from build123d import *

# Parameters (mm, degrees)
F1_DEPTH = 12
F3_DEPTH = 1
F4_R     = 1
F5_R     = 1.75
F6_DEPTH = 11.8
F7_R     = 2.25
F8_DEPTH = 4.8


with BuildPart() as f1:
    # F0 (on Front) → F1 (new body)
    with BuildSketch(Plane.XZ):
        with BuildLine():
            ThreePointArc((1, 3.872983), (0, -4), (-1, 3.872983))
            Line((-1, 3.872983), (-1, 14.872983))
            Line((-1, 14.872983), (-5, 14.872983))
            Line((-5, 14.872983), (-5, 6.244998))
            ThreePointArc((-5, 6.244998), (0, -8), (5, 6.244998))
            Line((5, 6.244998), (5, 14.872983))
            Line((5, 14.872983), (1, 14.872983))
            Line((1, 14.872983), (1, 3.872983))
        make_face()
    extrude(amount=F1_DEPTH)

    # F2 (on face) → F3 (join)
    with BuildSketch(Plane.XZ.offset(12)):
        with BuildLine():
            ThreePointArc((1, 3.872983), (0, -4), (-1, 3.872983))
            Line((-1, 3.872983), (-1, 5.408327))
            ThreePointArc((-1, 5.408327), (0, -5.5), (1, 5.408327))
            Line((1, 5.408327), (1, 3.872983))
        make_face()
    extrude(amount=F3_DEPTH)

    # F4
    f4_edges = [f1.edges().sort_by_distance(p)[0] for p in [
        (-1, -6.5, 3.872983),
        (1, -6.5, 3.872983),
    ]]
    fillet(f4_edges, radius=F4_R)

    # F5 (on face) → F6 (cut)
    with BuildSketch(Plane(origin=(-5, 0, 0), x_dir=(0, -1, 0), z_dir=(-1, 0, 0))):
        with Locations((6, 9.744998)):
            Circle(F5_R)
    extrude(amount=-F6_DEPTH, mode=Mode.SUBTRACT)

    # F7 (on face) → F8 (cut)
    with BuildSketch(Plane(origin=(-5, 0, 0), x_dir=(0, -1, 0), z_dir=(-1, 0, 0))):
        with Locations((6, 9.744998)):
            Circle(F7_R)
    extrude(amount=-F8_DEPTH, mode=Mode.SUBTRACT)


solid = f1.part
Part model, mm, in its own coordinate system. A direction names the side the tool comes from. Give positions to 0.01 mm unless a question says otherwise; leave off trailing zeros. Order: outer loops, then holes, each group sorted by start corner. A loop starts at its lowest first (then second) coordinate and runs counter-clockwise, first axis right, second up. Notation, with made-up numbers: (16.25, 8) - (34.25, 8) arc R21 cw to (34.25, 31) - close; hole circle Ø10 at (83, 63.5). An arc over 180 degrees is marked (long way). Use a Markdown table: item, result.
1) Flat gauge pins, fed straight in: P1, Ø4, axis at x = 3, z = 0, coming from the +Y side; P2, Ø2.5, axis at y = -5, z = 12, coming from the -X side; P3, Ø5, axis at y = -6, z = 9.74, coming from the +X side; P4, Ø2, axis at x = -1.5, z = 7.5, coming from the -Y side. Where does each tip first touch, or does it go through?
Checked values:
| item | result |
|---|---|
| P1 | y = 0 |
| P2 | x = -5 |
| P3 | x = 5 |
| P4 | y = -12 |
2) Probe L1, parallel to X at y = -6.25, z = 0; L2, parallel to Z at x = 3.6, y = -6 (3 decimals); L3, parallel to Z at x = 2.25, y = -6 (3 decimals). List the from-to ranges inside material, lowest first. Write a range as from..to.
Checked values:
| item | result |
|---|---|
| L1 | -8..-4, 4..8 |
| L2 | -7.144..-1.744, 1.744..7.995, 11.495..14.873 |
| L3 | -7.677..-3.307, 3.307..7.995, 11.495..14.873 |
3) 3-axis set-ups, long thin cutter, end or side, ignore diameter. For faces 1 (the flat face through (5, -4.6, 11.5)), 2 (the flat face through (-5, -5, 12)), 3 (the flat face through (1, -8, 10)), 4 (the cylindrical face through (1.168, -6.409, 4.028)): which of +Z, -Z, +X, -X, +Y, -Y reach the whole face in a straight line?
Checked values:
| item | result |
|---|---|
| face 1 | +Z, +X, +Y, -Y |
| face 2 | +Z, -X, +Y, -Y |
| face 3 | +Z, +Y, -Y |
| face 4 | +Y, -Y |
4) Saw through at D-D on x = 4.5. List the corners of the cut face in (y, z) (3 decimals).
Checked values:
| item | result |
|---|---|
| outline | (-13, -3.162) - (-12, -3.162) - (-12, -6.614) - (0, -6.614) - (0, 14.873) - (-12, 14.873) - (-12, 3.162) - (-13, 3.162) - close; hole circle Ø3.5 at (-6, 9.745) |
5) Saw through at C-C on y = -6. List the corners of the cut face in (x, z) (3 decimals), plus the area to 3 significant figures.
Checked values:
| item | result |
|---|---|
| outline | (-5, 6.245) arc R8 ccw (long way) to (5, 6.245) - (5, 7.995) - (1, 7.995) - (1, 4.583) arc R1 ccw to (1.6, 3.666) arc R4 cw (long way) to (-1.6, 3.666) arc R1 ccw to (-1, 4.583) - (-1, 7.495) - (-5, 7.495) - close; (-5, 11.995) - (-1, 11.995) - (-1, 14.873) - (-5, 14.873) - close; (1, 11.495) - (5, 11.495) - (5, 14.873) - (1, 14.873) - close |
| area | 171 mm² |
6) Saw through at B-B on x = -3.5. Count the separate pieces of the cut face and the enclosed holes in it, plus the area to 3 significant figures.
Checked values:
| item | result |
|---|---|
| separate pieces | 2 |
| enclosed holes | 1 |
| area | 207 mm² |
7) Saw through at A-A on z = 0. List the corners of the cut face in (x, y).
Checked values:
| item | result |
|---|---|
| outline | (-8, -12) - (-5.5, -12) - (-5.5, -13) - (-4, -13) - (-4, 0) - (-8, 0) - close; (4, -13) - (5.5, -13) - (5.5, -12) - (8, -12) - (8, 0) - (4, 0) - close |
8) Two-plate mould, pull along Y, no slides. Class faces 5 (the cylindrical face through (2.972, -5.621, 8.037)), 6 (the flat face through (-2, 0, 4)), 7 (the cylindrical face through (-0.228, -12.493, -5.495)): +Y half, -Y half, draft (parallel to the pull), parting line (faces both ways), or undercut.
Checked values:
| item | result |
|---|---|
| face 5 | undercut |
| face 6 | +Y half |
| face 7 | draft |
